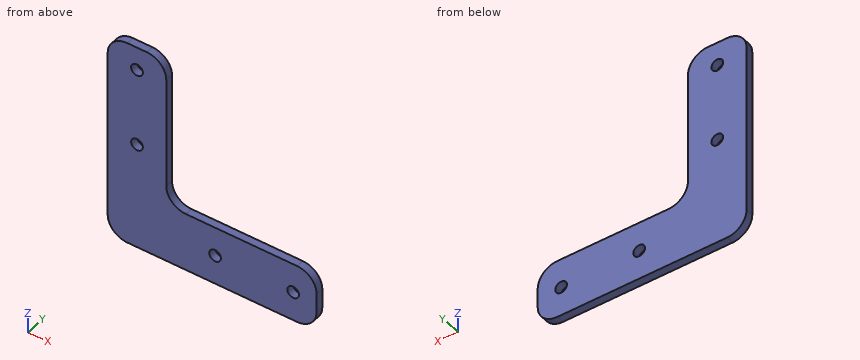
```python
from build123d import *

# Parameters (mm, degrees)
SKETCH1_R           = 1.5
BOSS_EXTRUDE1_DEPTH = 2
FILLET1_R           = 5


with BuildPart() as part:
    # Sketch1 → Boss-Extrude1 (new body)
    with BuildSketch(Plane(origin=(0, 0, 0), x_dir=(1, 0, 0), z_dir=(0, 1, 0))):
        Polygon((7.5, -7.5), (7.5, -46), (-7.5, -46), (-7.5, 7.5), (46, 7.5), (46, -7.5), align=None)
        with Locations((0, -40)):
            Circle(SKETCH1_R, mode=Mode.SUBTRACT)
        with Locations((0, -20)):
            Circle(SKETCH1_R, mode=Mode.SUBTRACT)
        with Locations((20, 0)):
            Circle(SKETCH1_R, mode=Mode.SUBTRACT)
        with Locations((40, 0)):
            Circle(SKETCH1_R, mode=Mode.SUBTRACT)
    extrude(amount=BOSS_EXTRUDE1_DEPTH)

    # Fillet1
    fillet1_edges = [part.edges().sort_by_distance(p)[0] for p in [
        (7.5, 1, 7.5),
        (7.5, 1, 46),
        (-7.5, 1, 46),
        (-7.5, 1, -7.5),
        (46, 1, -7.5),
        (46, 1, 7.5),
    ]]
    fillet(fillet1_edges, radius=FILLET1_R)


solid = part.part
```
Work out the finished part from the listing and answer in its coordinate system (mm). Round coordinates to 2 decimals unless told otherwise and drop trailing zeros. Order: outer loops, then holes, each group sorted by start corner. A loop starts at its lowest first (then second) coordinate and runs counter-clockwise, first axis right, second up.
Q1. Find the intervals of material crossed by line 1 along X through (y, z) = (1.4, 0); line 2 along Z through (x, y) = (40, 1.4), in increasing order.
Solution:
line 1: x = -7.5 to 18.5, 21.5 to 38.5, 41.5 to 46
line 2: z = -7.5 to -1.5, 1.5 to 7.5
Q2. A cutting plane is placed at B-B, the plane y = 1.5. Determine the outline of the cut face in (x, z).
Solution:
outline: (-7.5, -2.5) arc R5 ccw to (-2.5, -7.5) - (41, -7.5) arc R5 ccw to (46, -2.5) - (46, 2.5) arc R5 ccw to (41, 7.5) - (12.5, 7.5) arc R5 cw to (7.5, 12.5) - (7.5, 41) arc R5 ccw to (2.5, 46) - (-2.5, 46) arc R5 ccw to (-7.5, 41) - close; hole circle Ø3 at (0, 20); hole circle Ø3 at (0, 40); hole circle Ø3 at (20, 0); hole circle Ø3 at (40, 0)
Q3. Given pin 1 Ø2.5 at (x, z) = (0, 40) entering from -Y; pin 2 Ø0.6 at (x, y) = (22.5, 0.5) entering from +Z, each flat-ended and moving along its own axis, determine where each tip first touches the part or whether it passes through.
Solution:
pin 1: passes through
pin 2: stops at z = 7.5
Q4. A cutting plane is placed at A-A, the plane x = 40. Determine the outline of the cut face in (y, z).
Solution:
outline: (0, -7.5) - (2, -7.5) - (2, -1.5) - (0, -1.5) - close; (0, 1.5) - (2, 1.5) - (2, 7.5) - (0, 7.5) - close
Q5. A cutting plane is placed at C-C, the plane z = 0. Determine the outline of the cut face in (x, y).
Solution:
outline: (-7.5, 0) - (18.5, 0) - (18.5, 2) - (-7.5, 2) - close; (21.5, 0) - (38.5, 0) - (38.5, 2) - (21.5, 2) - close; (41.5, 0) - (46, 0) - (46, 2) - (41.5, 2) - close
Q6. A cutting plane is placed at D-D, the plane x = 0. Determine the outline of the cut face in (y, z).
Solution:
outline: (0, -7.5) - (2, -7.5) - (2, 18.5) - (0, 18.5) - close; (0, 21.5) - (2, 21.5) - (2, 38.5) - (0, 38.5) - close; (0, 41.5) - (2, 41.5) - (2, 46) - (0, 46) - close
